Part model, mm, in its own coordinate system. A direction names the side the tool comes from. Give positions to 0.01 mm unless a question says otherwise; leave off trailing zeros. Order: outer loops, then holes, each group sorted by start corner. A loop starts at its lowest first (then second) coordinate and runs counter-clockwise, first axis right, second up. Notation, with made-up numbers: M 54.5,25 L 98.5,25 A31 cw 98.5,64 Z; hole C -12.5,-39.75 d10. An arc over 180 degrees is marked long. Answer as a JSON object with one key per item and string values.
from build123d import *

# Parameters (mm, degrees)
ESQUISSE1_W                = 48
ESQUISSE1_H                = 24
EXTRUSION1_DEPTH           = 7.5
CONG_2_R                   = 5
CONG_5_R                   = 1
CONG_6_R                   = 1
ESQUISSE4_W                = 0.5
ESQUISSE4_H                = 18.982849842
EXTRUSION2_DEPTH           = 0.5
ESQUISSE5_R                = 0.25
EXTRUSION3_DEPTH           = 0.5
CHANFREIN1_SIZE            = 1
ESQUISSE10_R               = 2.5
EXTRUSION8_DEPTH           = 0.5
EXTRUSION8_DRAFT           = -45
ESQUISSE12_R               = 1.5
EXTRUSION9_DEPTH           = 0.5
EXTRUSION9_DRAFT           = -45
EXTRUSION9_PROFILE_2_DEPTH = 0.5
EXTRUSION9_PROFILE_2_DRAFT = -45
EXTRUSION9_PROFILE_3_DEPTH = 0.5
EXTRUSION9_PROFILE_3_DRAFT = -45
EXTRUSION9_PROFILE_4_DEPTH = 0.5
EXTRUSION9_PROFILE_4_DRAFT = -45
EXTRUSION9_PROFILE_5_DEPTH = 0.5
EXTRUSION9_PROFILE_5_DRAFT = -45
EXTRUSION9_PROFILE_6_DEPTH = 0.5
EXTRUSION9_PROFILE_6_DRAFT = -45


with BuildPart() as part:
    # Esquisse1 → Extrusion1 (new body)
    with BuildSketch(Plane(origin=(0, 0, 0), x_dir=(1, 0, 0), z_dir=(0, 1, 0))):
        with Locations((24, 12)):
            Rectangle(ESQUISSE1_W, ESQUISSE1_H)
    extrude(amount=EXTRUSION1_DEPTH)

    # Congé2
    cong_2_edges = [part.edges().sort_by_distance(p)[0] for p in [
        (0, 3.75, -24),
        (48, 3.75, -24),
        (48, 3.75, 0),
        (0, 3.75, 0),
    ]]
    fillet(cong_2_edges, radius=CONG_2_R)

    # Congé5
    cong_5_edges = [part.edges().sort_by_distance(p)[0] for p in [
        (48, 7.5, -12),
        (24, 7.5, 0),
        (0, 7.5, -12),
        (24, 7.5, -24),
        (1.464466094, 7.5, -22.535533906),
        (1.464466094, 7.5, -1.464466094),
        (46.535533906, 7.5, -22.535533906),
        (46.535533906, 7.5, -1.464466094),
    ]]
    fillet(cong_5_edges, radius=CONG_5_R)

    # Congé6
    cong_6_edges = [part.edges().sort_by_distance(p)[0] for p in [
        (48, 0, -12),
        (0, 0, -12),
        (24, 0, -24),
        (24, 0, 0),
        (1.464466094, 0, -22.535533906),
        (1.464466094, 0, -1.464466094),
        (46.535533906, 0, -22.535533906),
        (46.535533906, 0, -1.464466094),
    ]]
    fillet(cong_6_edges, radius=CONG_6_R)

    # Esquisse4 → Extrusion2 (cut)
    with BuildSketch(Plane(origin=(0, 7.5, 0), x_dir=(1, 0, 0), z_dir=(0, 1, 0))):
        with Locations((24, 12)):
            Rectangle(ESQUISSE4_W, ESQUISSE4_H)
    extrude(amount=-EXTRUSION2_DEPTH, mode=Mode.SUBTRACT)

    # Esquisse5 → Extrusion3 (cut)
    with BuildSketch(Plane(origin=(0, 7.5, 0), x_dir=(1, 0, 0), z_dir=(0, 1, 0))):
        with Locations((24, 21.491424921)):
            Circle(ESQUISSE5_R)
        with Locations((24, 2.508575079)):
            Circle(ESQUISSE5_R)
    extrude(amount=-EXTRUSION3_DEPTH, mode=Mode.SUBTRACT)

    # Chanfrein1
    # the kernel refuses this chamfer: 1 mm, written as the material it takes off along each edge
    with BuildSketch(Plane(origin=(24, 7.5, -21.491424921), x_dir=(1, 0, 0), z_dir=(0, 0, 1))) as chanfrein1_piece_1_section:
        Polygon((0.25 + CHANFREIN1_SIZE, 0), (0.25, -CHANFREIN1_SIZE), (0.25, 0), align=None)
    chanfrein1_piece_1 = revolve(axis=Axis((24, 7.5, -21.491424921), (0, 1, 0)), revolution_arc=180, mode=Mode.PRIVATE)
    chanfrein1_piece_1 = split(chanfrein1_piece_1, bisect_by=Plane(origin=(24, 7, -21.964580549), z_dir=(0, 1, 0)), keep=Keep.TOP, mode=Mode.PRIVATE)
    add(chanfrein1_piece_1, mode=Mode.SUBTRACT)
    with BuildSketch(Plane(origin=(24.25, 7.5, -21.491424921), x_dir=(0.9996219169112968, 0.02749587661058651, 0), z_dir=(0, 0, 1))) as chanfrein1_piece_2_section:
        Polygon((CHANFREIN1_SIZE * 0.999621916911, -CHANFREIN1_SIZE * 0.0274958766106), (-CHANFREIN1_SIZE * 0.0274958766106, -CHANFREIN1_SIZE * 0.999621916911), (0, 0), align=None)
    chanfrein1_piece_2 = extrude(amount=18.982849842, mode=Mode.PRIVATE)
    chanfrein1_piece_2 = split(chanfrein1_piece_2, bisect_by=Plane(origin=(24.643401084, 7, -12), z_dir=(0, 1, 0)), keep=Keep.TOP, mode=Mode.PRIVATE)
    add(chanfrein1_piece_2, mode=Mode.SUBTRACT)
    with BuildSketch(Plane(origin=(24, 7.5, -2.508575079), x_dir=(-1, 0, 0), z_dir=(0, 0, -1))) as chanfrein1_piece_3_section:
        Polygon((0.25 + CHANFREIN1_SIZE, 0), (0.25, -CHANFREIN1_SIZE), (0.25, 0), align=None)
    chanfrein1_piece_3 = revolve(axis=Axis((24, 7.5, -2.508575079), (0, 1, 0)), revolution_arc=180, mode=Mode.PRIVATE)
    chanfrein1_piece_3 = split(chanfrein1_piece_3, bisect_by=Plane(origin=(24, 7, -2.035419451), z_dir=(0, 1, 0)), keep=Keep.TOP, mode=Mode.PRIVATE)
    add(chanfrein1_piece_3, mode=Mode.SUBTRACT)
    with BuildSketch(Plane(origin=(23.75, 7.5, -2.508575079), x_dir=(-0.9996219169112968, 0.02749587661058651, 0), z_dir=(0, 0, -1))) as chanfrein1_piece_4_section:
        Polygon((CHANFREIN1_SIZE * 0.999621916911, -CHANFREIN1_SIZE * 0.0274958766106), (-CHANFREIN1_SIZE * 0.0274958766106, -CHANFREIN1_SIZE * 0.999621916911), (0, 0), align=None)
    chanfrein1_piece_4 = extrude(amount=18.982849842, mode=Mode.PRIVATE)
    chanfrein1_piece_4 = split(chanfrein1_piece_4, bisect_by=Plane(origin=(23.356598916, 7, -12), z_dir=(0, 1, 0)), keep=Keep.TOP, mode=Mode.PRIVATE)
    add(chanfrein1_piece_4, mode=Mode.SUBTRACT)


with BuildPart() as extrusion8_tool:
    # Esquisse10 → Extrusion8 (with draft: the straight prism first)
    with BuildSketch(Plane(origin=(0, 7.5, 0), x_dir=(1, 0, 0), z_dir=(0, 1, 0))):
        with Locations((12, 12)):
            Circle(ESQUISSE10_R)
    extrude(amount=-EXTRUSION8_DEPTH)
    # Extrusion8: the draft: its side faces are tilted about the plane it starts from
    extrusion8_sides = [extrusion8_tool.faces().sort_by_distance(p)[0] for p in [
        (9.5, 7.25, -12),
    ]]
    draft(extrusion8_sides, Plane(origin=(0, 7.5, 0), x_dir=(1, 0, 0), z_dir=(0, 1, 0)), EXTRUSION8_DRAFT)


with BuildPart() as part_1:
    add(part.part)

    # Extrusion8: cut by extrusion8_tool
    add(extrusion8_tool.part, mode=Mode.SUBTRACT)


with BuildPart() as extrusion9_tool:
    # Esquisse12 → Extrusion9 (with draft: the straight prism first)
    with BuildSketch(Plane(origin=(0, 7.5, 0), x_dir=(1, 0, 0), z_dir=(0, 1, 0))):
        with Locations((30.25, 17)):
            Circle(ESQUISSE12_R)
    extrude(amount=-EXTRUSION9_DEPTH)
    # Extrusion9: the draft: its side faces are tilted about the plane it starts from
    extrusion9_sides = [extrusion9_tool.faces().sort_by_distance(p)[0] for p in [
        (28.75, 7.25, -17),
    ]]
    draft(extrusion9_sides, Plane(origin=(0, 7.5, 0), x_dir=(1, 0, 0), z_dir=(0, 1, 0)), EXTRUSION9_DRAFT)


with BuildPart() as part_2:
    add(part_1.part)

    # Extrusion9: cut by extrusion9_tool
    add(extrusion9_tool.part, mode=Mode.SUBTRACT)


with BuildPart() as extrusion9_profile_2_tool:
    # Esquisse12 → Extrusion9 profile 2 (with draft: the straight prism first)
    with BuildSketch(Plane(origin=(0, 7.5, 0), x_dir=(1, 0, 0), z_dir=(0, 1, 0))):
        with Locations((36.125, 17)):
            Circle(ESQUISSE12_R)
    extrude(amount=-EXTRUSION9_PROFILE_2_DEPTH)
    # Extrusion9 profile 2: the draft: its side faces are tilted about the plane it starts from
    extrusion9_profile_2_sides = [extrusion9_profile_2_tool.faces().sort_by_distance(p)[0] for p in [
        (34.625, 7.25, -17),
    ]]
    draft(extrusion9_profile_2_sides, Plane(origin=(0, 7.5, 0), x_dir=(1, 0, 0), z_dir=(0, 1, 0)), EXTRUSION9_PROFILE_2_DRAFT)


with BuildPart() as part_3:
    add(part_2.part)

    # Extrusion9 profile 2: cut by extrusion9_profile_2_tool
    add(extrusion9_profile_2_tool.part, mode=Mode.SUBTRACT)


with BuildPart() as extrusion9_profile_3_tool:
    # Esquisse12 → Extrusion9 profile 3 (with draft: the straight prism first)
    with BuildSketch(Plane(origin=(0, 7.5, 0), x_dir=(1, 0, 0), z_dir=(0, 1, 0))):
        with Locations((42, 17)):
            Circle(ESQUISSE12_R)
    extrude(amount=-EXTRUSION9_PROFILE_3_DEPTH)
    # Extrusion9 profile 3: the draft: its side faces are tilted about the plane it starts from
    extrusion9_profile_3_sides = [extrusion9_profile_3_tool.faces().sort_by_distance(p)[0] for p in [
        (40.5, 7.25, -17),
    ]]
    draft(extrusion9_profile_3_sides, Plane(origin=(0, 7.5, 0), x_dir=(1, 0, 0), z_dir=(0, 1, 0)), EXTRUSION9_PROFILE_3_DRAFT)


with BuildPart() as part_4:
    add(part_3.part)

    # Extrusion9 profile 3: cut by extrusion9_profile_3_tool
    add(extrusion9_profile_3_tool.part, mode=Mode.SUBTRACT)


with BuildPart() as extrusion9_profile_4_tool:
    # Esquisse12 → Extrusion9 profile 4 (with draft: the straight prism first)
    with BuildSketch(Plane(origin=(0, 7.5, 0), x_dir=(1, 0, 0), z_dir=(0, 1, 0))):
        with Locations((30.25, 7)):
            Circle(ESQUISSE12_R)
    extrude(amount=-EXTRUSION9_PROFILE_4_DEPTH)
    # Extrusion9 profile 4: the draft: its side faces are tilted about the plane it starts from
    extrusion9_profile_4_sides = [extrusion9_profile_4_tool.faces().sort_by_distance(p)[0] for p in [
        (28.75, 7.25, -7),
    ]]
    draft(extrusion9_profile_4_sides, Plane(origin=(0, 7.5, 0), x_dir=(1, 0, 0), z_dir=(0, 1, 0)), EXTRUSION9_PROFILE_4_DRAFT)


with BuildPart() as part_5:
    add(part_4.part)

    # Extrusion9 profile 4: cut by extrusion9_profile_4_tool
    add(extrusion9_profile_4_tool.part, mode=Mode.SUBTRACT)


with BuildPart() as extrusion9_profile_5_tool:
    # Esquisse12 → Extrusion9 profile 5 (with draft: the straight prism first)
    with BuildSketch(Plane(origin=(0, 7.5, 0), x_dir=(1, 0, 0), z_dir=(0, 1, 0))):
        with Locations((36.125, 7)):
            Circle(ESQUISSE12_R)
    extrude(amount=-EXTRUSION9_PROFILE_5_DEPTH)
    # Extrusion9 profile 5: the draft: its side faces are tilted about the plane it starts from
    extrusion9_profile_5_sides = [extrusion9_profile_5_tool.faces().sort_by_distance(p)[0] for p in [
        (34.625, 7.25, -7),
    ]]
    draft(extrusion9_profile_5_sides, Plane(origin=(0, 7.5, 0), x_dir=(1, 0, 0), z_dir=(0, 1, 0)), EXTRUSION9_PROFILE_5_DRAFT)


with BuildPart() as part_6:
    add(part_5.part)

    # Extrusion9 profile 5: cut by extrusion9_profile_5_tool
    add(extrusion9_profile_5_tool.part, mode=Mode.SUBTRACT)


with BuildPart() as extrusion9_profile_6_tool:
    # Esquisse12 → Extrusion9 profile 6 (with draft: the straight prism first)
    with BuildSketch(Plane(origin=(0, 7.5, 0), x_dir=(1, 0, 0), z_dir=(0, 1, 0))):
        with Locations((42, 7)):
            Circle(ESQUISSE12_R)
    extrude(amount=-EXTRUSION9_PROFILE_6_DEPTH)
    # Extrusion9 profile 6: the draft: its side faces are tilted about the plane it starts from
    extrusion9_profile_6_sides = [extrusion9_profile_6_tool.faces().sort_by_distance(p)[0] for p in [
        (40.5, 7.25, -7),
    ]]
    draft(extrusion9_profile_6_sides, Plane(origin=(0, 7.5, 0), x_dir=(1, 0, 0), z_dir=(0, 1, 0)), EXTRUSION9_PROFILE_6_DRAFT)


with BuildPart() as part_7:
    add(part_6.part)

    # Extrusion9 profile 6: cut by extrusion9_profile_6_tool
    add(extrusion9_profile_6_tool.part, mode=Mode.SUBTRACT)


solid = part_7.part
1. Which spindle directions (+Z, -Z, +X, -X, +Y, -Y) get a long thin tool onto all of the face, cutting with end or side? Do faces 1 (the flat face through (24, 4, 0)), 2 (the flat face through (30, 7, -7)). Say none if no direction does.
Worked answers:
{"face 1": "+Z, +X, -X, +Y, -Y", "face 2": "+Y"}
2. Probe line 1 along Z through (x, y) = (31, 7.25); line 2 along Y through (x, z) = (23.5, -6.5); line 3 along Z through (x, y) = (33, 7.25). List the from-to ranges inside material, lowest first.
Worked answers:
{"line 1": "z = -23.66 to -18, -16 to -8, -6 to -0.34", "line 2": "y = 0 to 7", "line 3": "z = -23.66 to -0.34"}
3. Two-plate mould, pull along X, no slides. Class faces 3 (the cylindrical face through (1, 4, -22)), 4 (the cylindrical face through (23.734, 7.215, -23.699)), 5 (the flat face through (42, 7, -17)): +X half, -X half, draft (parallel to the pull), parting line (faces both ways), or undercut.
Worked answers:
{"face 3": "-X half", "face 4": "draft", "face 5": "undercut"}
4. Pin check, flat tips, straight feed: P1, Ø1, axis at x = 36, z = -17, coming from the +Y side; P2, Ø1.6, axis at x = 30.5, z = -17, coming from the +Y side; P3, Ø2, axis at x = 30.5, z = -7.5, coming from the +Y side. Stop position of each tip, or through.
Worked answers:
{"P1": "stops at y = 7", "P2": "stops at y = 7.05", "P3": "stops at y = 7.5"}
5. Cut at B-B on z = -17. Give the cut face in (x, y) (3 decimals).
Worked answers:
{"outline": "M 0,1 A1 ccw 1,0 L 47,0 A1 ccw 48,1 L 48,6.5 A1 ccw 47,7.5 L 43.5,7.5 L 43,7 L 41,7 L 40.5,7.5 L 37.625,7.5 L 37.125,7 L 35.125,7 L 34.625,7.5 L 31.75,7.5 L 31.25,7 L 29.25,7 L 28.75,7.5 L 25.25,7.5 L 24.75,7 L 23.25,7 L 22.75,7.5 L 1,7.5 A1 ccw 0,6.5 Z"}
6. Cut at A-A on x = 42. Give the cut face in (y, z).
Worked answers:
{"outline": "M 0,-23 A1 ccw 1,-24 L 6.5,-24 A1 ccw 7.5,-23 L 7.5,-18.5 L 7,-18 L 7,-16 L 7.5,-15.5 L 7.5,-8.5 L 7,-8 L 7,-6 L 7.5,-5.5 L 7.5,-1 A1 ccw 6.5,0 L 1,0 A1 ccw 0,-1 Z"}
7. Cut at C-C on x = 12. Give the cut face in (y, z).
Worked answers:
{"outline": "M 0,-23 A1 ccw 1,-24 L 6.5,-24 A1 ccw 7.5,-23 L 7.5,-14.5 L 7,-14 L 7,-10 L 7.5,-9.5 L 7.5,-1 A1 ccw 6.5,0 L 1,0 A1 ccw 0,-1 Z"}
